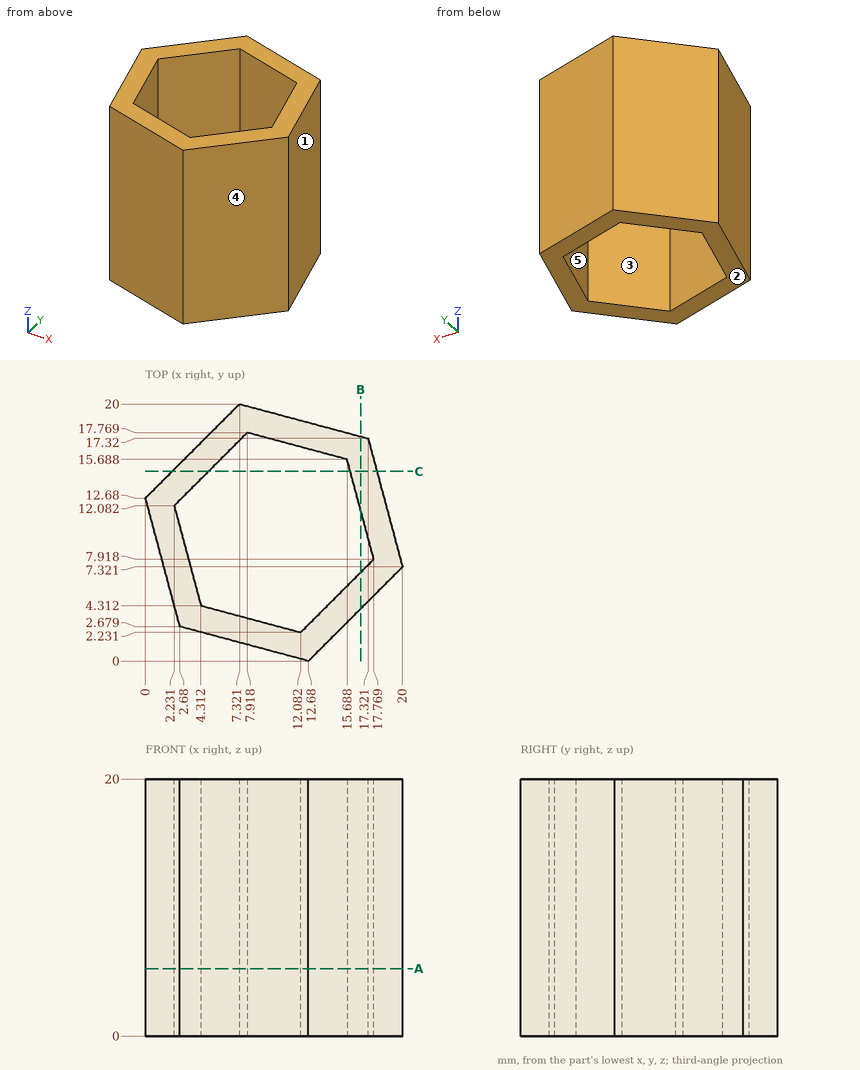
Print and shaded views of the part. All mm, measured from the part's lowest x, y and z. A direction names the side the tool comes from. Give positions to 0.01 mm unless a question says otherwise; leave off trailing zeros. Loops run counter-clockwise (first coordinate to the right, second up) from the corner with the lowest first, then second, coordinate; pieces in that order, holes last. Notation, with made-up numbers: (-26.75, -29) - (15.25, -29) arc R31 ccw to (15.25, -1) - close; hole circle Ø5 at (39, 74). An arc over 180 degrees is marked (long way). One line per item, written item: value. Start each with the question number.
1. Slice it at A-A (z = 5.25). List the corners of the cut face in (x, y).
2. Which spindle directions (+Z, -Z, +X, -X, +Y, -Y) get a long thin tool onto all of the face, cutting with end or side? Do the marked faces 4 and 5. Say none if no direction does.
3. Slice it at C-C (y = 14.75). List the corners of the cut face in (x, z).
4. Slice it at B-B (x = 16.75). List the corners of the cut face in (y, z).
5. Pull direction X, two halves, no side cores. Call the marked faces 1, 2 and 3: pulls with the +X half, pulls with the -X half, needs draft (parallel to the pull), parting line crosses it, or undercut.
6. Pin check, flat tips, straight feed: pin 1 (1.5 mm diameter, centred on x = 10, z = 2.5, fed in from -Y); pin 2 (4 mm diameter, centred on y = 9, z = 10, fed in from -X). Stop position of each tip, or through.
7. Probe L1, parallel to Y at x = 12.75, z = 7.25 (1 decimal); L2, parallel to Y at x = 11.5, z = 8.5 (1 decimal); L3, parallel to X at y = 10.5, z = 1.5 (1 decimal). List the from-to ranges inside material, lowest first. Write a range as from..to.
Solution:
1. outline: (0, 12.68) - (2.68, 2.68) - (12.68, 0) - (20, 7.32) - (17.32, 17.32) - (7.32, 20) - close; hole (2.23, 12.08) - (4.31, 4.31) - (12.08, 2.23) - (17.77, 7.92) - (15.69, 15.69) - (7.92, 17.77) - close
2. face 4: +Z, -Z, +X, -Y
2. face 5: +Z, -Z
3. outline: (2.07, 0) - (4.9, 0) - (4.9, 20) - (2.07, 20) - close; (15.94, 0) - (18.01, 0) - (18.01, 20) - (15.94, 20) - close
4. outline: (4.07, 0) - (6.9, 0) - (6.9, 20) - (4.07, 20) - close; (11.72, 0) - (17.47, 0) - (17.47, 20) - (11.72, 20) - close
5. face 1: pulls with the +X half
5. face 2: needs draft
5. face 3: undercut
6. pin 1: stops at y = 0.52
6. pin 2: stops at x = 0.45
7. L1: y = 0.1..2.9, 16.5..18.5
7. L2: y = 0.3..2.4, 16.8..18.9
7. L3: x = 0.6..2.7, 17.1..19.1
